from build123d import *

# Parameters (mm, degrees)
SKETCH_1_R          = 1.55
SKETCH_1_W          = 37
SKETCH_1_H          = 7
EXTRUDE_1_DEPTH     = 3
SKETCH_2_R          = 2
CUT_EXTRUDE_1_DEPTH = 10
EXTRUDE_START       = -3
SKETCH_3_R          = 1.55
EXTRUDE_2_DEPTH     = 3
FILLET_1_R          = 1


with BuildPart() as part:
    # 草图1 → 凸台-拉伸1 (new body)
    # profile 1 of 2: a face of its own
    with BuildSketch(Plane(origin=(0, 0, 0), x_dir=(0, 0, -1), z_dir=(1, 0, 0))):
        Polygon((28, -59.25), (12.5, -39.75), (-12.5, -39.75), (-28, -59.25), (-28, -69.25), (-20.5, -69.25), (-15.881197846, -61.25), (15.881197846, -61.25), (20.5, -69.25), (28, -69.25), align=None)
        with Locations((-24.5, -66.75)):
            Circle(SKETCH_1_R, mode=Mode.SUBTRACT)
        with Locations((24.5, -66.75)):
            Circle(SKETCH_1_R, mode=Mode.SUBTRACT)
    # profile 2 of 2: a face of its own
    with BuildSketch(Plane(origin=(0, 0, 0), x_dir=(0, 0, -1), z_dir=(1, 0, 0))):
        Polygon((-12.5, -39.75), (12.5, -39.75), (12.5, -28.75), (12.5, -13.75), (12.5, 25.75), (16.5, 28.059401077), (16.5, 37.440598923), (12.5, 39.75), (-12.5, 39.75), (-16.5, 37.440598923), (-16.5, 28.059401077), (-12.5, 25.75), (-12.5, -13.75), (-52.5, -13.75), (-52.5, -28.75), (-12.5, -28.75), align=None)
        with Locations((-30, -21.25)):
            Rectangle(SKETCH_1_W, SKETCH_1_H, mode=Mode.SUBTRACT)
        with Locations((-8, -33.75)):
            Circle(SKETCH_1_R, mode=Mode.SUBTRACT)
        with BuildLine():
            ThreePointArc((2.605, -35.095), (2.310642315, -35.805642315), (1.6, -36.1))
            Line((1.6, -36.1), (-1.6, -36.1))
            ThreePointArc((-1.6, -36.1), (-2.605, -35.095), (-1.6, -34.09))
            Line((-1.6, -34.09), (-1.6, -17.91))
            ThreePointArc((-1.6, -17.91), (-2.605, -16.905), (-1.6, -15.9))
            Line((-1.6, -15.9), (1.6, -15.9))
            ThreePointArc((1.6, -15.9), (2.310642315, -16.194357685), (2.605, -16.905))
            ThreePointArc((2.605, -16.905), (2.310642315, -17.615642315), (1.6, -17.91))
            Line((1.6, -17.91), (1.6, -34.09))
            ThreePointArc((1.6, -34.09), (2.310642315, -34.384357685), (2.605, -35.095))
        make_face(mode=Mode.SUBTRACT)
        with Locations((8, -33.75)):
            Circle(SKETCH_1_R, mode=Mode.SUBTRACT)
        with BuildLine():
            ThreePointArc((2.605, 4.905), (2.310642315, 4.194357685), (1.6, 3.9))
            Line((1.6, 3.9), (-1.6, 3.9))
            ThreePointArc((-1.6, 3.9), (-2.605, 4.905), (-1.6, 5.91))
            Line((-1.6, 5.91), (-1.6, 22.09))
            ThreePointArc((-1.6, 22.09), (-2.605, 23.095), (-1.6, 24.1))
            Line((-1.6, 24.1), (1.6, 24.1))
            ThreePointArc((1.6, 24.1), (2.310642315, 23.805642315), (2.605, 23.095))
            ThreePointArc((2.605, 23.095), (2.310642315, 22.384357685), (1.6, 22.09))
            Line((1.6, 22.09), (1.6, 5.91))
            ThreePointArc((1.6, 5.91), (2.310642315, 5.615642315), (2.605, 4.905))
        make_face(mode=Mode.SUBTRACT)
        with BuildLine():
            Line((10.49, 31.05), (-10.49, 31.05))
            ThreePointArc((-10.49, 31.05), (-11.495, 30.045), (-12.5, 31.05))
            Line((-12.5, 31.05), (-12.5, 34.45))
            ThreePointArc((-12.5, 34.45), (-11.495, 35.455), (-10.49, 34.45))
            Line((-10.49, 34.45), (10.49, 34.45))
            ThreePointArc((10.49, 34.45), (11.495, 35.455), (12.5, 34.45))
            Line((12.5, 34.45), (12.5, 31.05))
            ThreePointArc((12.5, 31.05), (11.495, 30.045), (10.49, 31.05))
        make_face(mode=Mode.SUBTRACT)
    extrude(amount=EXTRUDE_1_DEPTH)

    # 草图2 → 切除-拉伸1 (cut)
    with BuildSketch(Plane(origin=(3, 0, 0), x_dir=(0, 0, -1), z_dir=(1, 0, 0))):
        with Locations((15.3, -50.25)):
            Circle(SKETCH_2_R)
        with Locations((-15.3, -50.25)):
            Circle(SKETCH_2_R)
        Polygon((33.5, -57.75), (33.5, -62.75), (25.5, -62.75), (25.5, -57.75), (25.5, -56.10483871), (33.5, -56.10483871), align=None)
        Polygon((-33.5, -62.75), (-25.5, -62.75), (-25.5, -57.75), (-25.5, -56.10483871), (-33.5, -56.10483871), (-33.5, -57.75), align=None)
        Polygon((12.725724403, -56.10483871), (2.5, -56.10483871), (2.5, -43.240217687), align=None)
        Polygon((-2.5, -56.10483871), (-2.5, -43.240217687), (-12.725724403, -56.10483871), align=None)
    extrude(amount=-CUT_EXTRUDE_1_DEPTH, mode=Mode.SUBTRACT)

    # 草图3 → 凸台-拉伸2 (add)
    # profile 1 of 4: a face of its own
    with BuildSketch(Plane(origin=(3, 0, 0), x_dir=(0, 0, -1), z_dir=(1, 0, 0)).offset(EXTRUDE_START)):
        with BuildLine():
            Line((-3.757359313, -27.75), (-11.605551275, -27.75))
            ThreePointArc((-11.605551275, -27.75), (-13.792647393, -37.680042771), (-3.757359313, -39.317764363))
            Line((-3.757359313, -39.317764363), (-3.757359313, -27.75))
        make_face()
        with Locations((-8, -33.75)):
            Circle(SKETCH_3_R, mode=Mode.SUBTRACT)
    # profile 2 of 4: a face of its own
    with BuildSketch(Plane(origin=(3, 0, 0), x_dir=(0, 0, -1), z_dir=(1, 0, 0)).offset(EXTRUDE_START)):
        with BuildLine():
            Line((11.605551275, -27.75), (3.757359313, -27.75))
            Line((3.757359313, -27.75), (3.757359313, -39.317764363))
            ThreePointArc((3.757359313, -39.317764363), (13.792647393, -37.680042771), (11.605551275, -27.75))
        make_face()
        with Locations((8, -33.75)):
            Circle(SKETCH_3_R, mode=Mode.SUBTRACT)
    # profile 3 of 4: a face of its own
    with BuildSketch(Plane(origin=(3, 0, 0), x_dir=(0, 0, -1), z_dir=(1, 0, 0)).offset(EXTRUDE_START)):
        with BuildLine():
            Line((-21.275623434, -50.790300449), (-16.121878581, -44.306556924))
            ThreePointArc((-16.121878581, -44.306556924), (-19.996939529, -46.516535247), (-21.275623434, -50.790300449))
        make_face()
    # profile 4 of 4: a face of its own
    with BuildSketch(Plane(origin=(3, 0, 0), x_dir=(0, 0, -1), z_dir=(1, 0, 0)).offset(EXTRUDE_START)):
        with BuildLine():
            Line((21.275623434, -50.790300449), (16.121878581, -44.306556924))
            ThreePointArc((16.121878581, -44.306556924), (19.996939529, -46.516535247), (21.275623434, -50.790300449))
        make_face()
    extrude(amount=EXTRUDE_2_DEPTH)

    # 圆角1
    fillet_1_edges = [part.edges().sort_by_distance(p)[0] for p in [
        (1.5, -17.75, 48.5),
        (1.5, -24.75, 48.5),
        (1.5, -24.75, 11.5),
        (1.5, -17.75, 11.5),
        (1.5, -62.75, -25.5),
        (1.5, -62.75, -28),
        (1.5, -56.10483871, 12.725724403),
        (1.5, -43.240217687, 2.5),
        (1.5, -56.10483871, 2.5),
        (1.5, -62.75, 28),
        (1.5, -62.75, 25.5),
        (1.5, -43.240217687, -2.5),
        (1.5, -56.10483871, -12.725724403),
        (1.5, -56.10483871, -2.5),
        (1.5, -69.25, -28),
        (1.5, -69.25, -20.5),
        (1.5, -61.25, -15.881197846),
        (1.5, -61.25, 15.881197846),
        (1.5, -69.25, 20.5),
        (1.5, -69.25, 28),
        (1.5, -28.75, 52.5),
        (1.5, -13.75, 52.5),
        (1.5, -13.75, 12.5),
    ]]
    fillet(fillet_1_edges, radius=FILLET_1_R)


solid = part.part
The model under review builds one solid part; all positions refer to its coordinate system, in mm. A direction names the side the tool comes from. Give positions to 0.01 mm unless a question says otherwise; leave off trailing zeros. Order: outer loops, then holes, each group sorted by start corner. A loop starts at its lowest first (then second) coordinate and runs counter-clockwise, first axis right, second up. Notation, with made-up numbers: M 32.25,-5.5 L 71.25,-5.5 A19 ccw 71.25,18.5 Z; hole C -38.75,-23 d10. An arc over 180 degrees is marked long. Use one line per item in the form item = value. Start each with the question number.
Item 1: We need section C-C on z = -8. Give the boundary of the cut face in (x, y), plus the area to 3 significant figures.
Item 2: For faces 4 (the flat face through (1.479, -42.06, -14.336)), 5 (the flat face through (1.48, 26.92, 14.53)), 6 (the flat face through (2, -59, -25.5)), 7 (the flat face through (1, -17.75, 30)), list the 3-axis set-ups (+Z, -Z, +X, -X, +Y, -Y) from which the entire face can be reached by the end or side of a thin tool; tool diameter is ignored.
Item 3: We need section B-B on y = 10. Give the boundary of the cut face in (x, z).
Item 4: The part is to be moulded in two halves that separate along Z. For faces 1 (the flat face through (1, 33, 16.5)), 2 (the flat face through (1.48, -65.3, 18.22)), 3 (the flat face through (1, -28.75, 32)), say which applies: pulls with the +Z half, pulls with the -Z half, needs draft (parallel to the pull), parting line crosses it, or undercut.
Item 5: We need section A-A on z = 29.5. Give the boundary of the cut face in (x, y).
Item 6: Insertion check: pin 1 Ø0.9 at (x, z) = (2, 2) entering from -Y; pin 2 Ø0.9 at (x, y) = (1, 33.5) entering from +Z; pin 3 Ø0.9 at (x, y) = (2, -52.5) entering from +Z. Each pin has a flat end and moves straight along its axis. Give the tip position at first contact, or say it passes through.
Item 7: To check wall thickness, follow line 1 along Z through (x, y) = (2.25, 20.5); line 2 along Z through (x, y) = (1.6, -66.75); line 3 along Y through (x, z) = (0.95, 38.5). State the ranges of each line that lie inside material, in increasing order. Write a range as from..to.
Item 8: We need section D-D on x = 1.2. Give the number of separate pieces and of enclosed holes in the cut face, plus the area to 3 significant figures.
Completed:
q1.outline = M 0,-61.25 L 3,-61.25 L 3,-56.1 L 0,-56.1 Z; M 0,-50.16 L 3,-50.16 L 3,-35.3 L 0,-35.3 Z; M 0,-32.2 L 3,-32.2 L 3,31.05 L 0,31.05 Z; M 0,34.45 L 3,34.45 L 3,39.75 L 0,39.75 Z
q1.area = 266 mm²
q2.face_4 = -Z, +X, -X
q2.face_5 = +Z, +X, -X
q2.face_6 = -Z, +X, -X, +Y
q2.face_7 = +X, -X
q3.outline = M 0,-12.5 L 3,-12.5 L 3,-1.6 L 0,-1.6 Z; M 0,1.6 L 3,1.6 L 3,12.5 L 0,12.5 Z
q4.face_1 = pulls with the +Z half
q4.face_2 = undercut
q4.face_3 = needs draft
q5.outline = M 0,-28.75 L 3,-28.75 L 3,-24.75 L 0,-24.75 Z; M 0,-17.75 L 3,-17.75 L 3,-13.75 L 0,-13.75 Z
q6.pin_1 = -61.25
q6.pin_2 = 16.5
q6.pin_3 = 22.99
q7.line_1 = -12.5..-1.6, 1.6..12.5
q7.line_2 = -28..-26.05, -22.95..-19.06, 19.06..22.95, 26.05..28
q7.line_3 = -28.75..-24.75, -17.75..-13.75
q8.separate_pieces = 1
q8.enclosed_holes = 12
q8.area = 3,100 mm²
